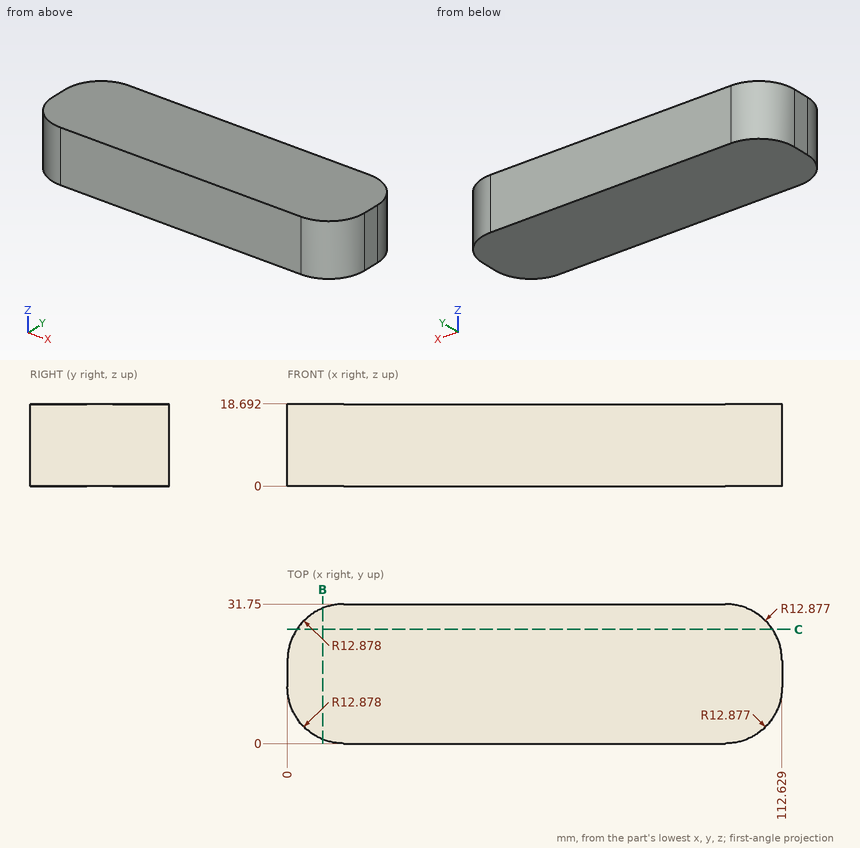
The figure shows three views and two pictorial views of one solid part (mm, origin at its lowest corner). Answer the questions. Coordinates: 2 decimals unless noted, no trailing zeros. Loops run counter-clockwise (first coordinate to the right, second up) from the corner with the lowest first, then second, coordinate; pieces in that order, holes last. Notation, with made-up numbers: (24, 82) - (31, 82) arc R24 cw to (31, 110) - close; hole circle Ø9 at (39.25, 22.25). An arc over 180 degrees is marked (long way). Answer in a Markdown table with one row per item.
Q1. Find section C-C on y = 26. Write down the section's boundary in (x, z), plus the area to 3 significant figures.
Here are the results:
| item | result |
|---|---|
| outline | (2.15, 0) - (110.48, 0) - (110.48, 18.69) - (2.15, 18.69) - close |
| area | 2,020 mm^2 |
Q2. Straight lines are drawn through the part: line 1 along X through (y, z) = (9.5, 1.5); line 2 along X through (y, z) = (4.5, 15.75); line 3 along Y through (x, z) = (11.5, 1.5). For each, find the intervals that lie inside material, in ascending order. Write a range as [from, to].
Here are the results:
| item | result |
|---|---|
| line 1 | x = [0.45, 112.18] |
| line 2 | x = [3.1, 109.53] |
| line 3 | y = [0.07, 31.68] |
Q3. Given P1, Ø1, axis at y = 27, z = 15.5, coming from the +X side; P2, Ø6, axis at y = 28, z = 5, coming from the -X side, each flat-ended and moving along its own axis, determine where each tip first touches the part or whether it passes through.
Here are the results:
| item | result |
|---|---|
| P1 | stops at x = 110.13 |
| P2 | stops at x = 1.55 |
Q4. Find section B-B on x = 8. Write down the section's boundary in (y, z).
Here are the results:
| item | result |
|---|---|
| outline | (0.96, 0) - (30.79, 0) - (30.79, 18.69) - (0.96, 18.69) - close |
